```python
from build123d import *

# Parameters (mm, degrees)
PAD_DEPTH = 6


with BuildPart() as part:
    # Sketch → Pad (new body)
    with BuildSketch(Plane.XY):
        with BuildLine():
            ThreePointArc((-202.000023, 6.75), (-208.750028, -1e-06), (-202.000021, -6.75))
            Line((-202.000021, -6.75), (201.999979, -6.75))
            ThreePointArc((201.999979, -6.75), (208.74998, 1e-06), (201.999977, 6.75))
            Line((-202.000023, 6.75), (201.999977, 6.75))
        make_face()
        with BuildLine():
            Line((-202, 5.25), (202, 5.25))
            ThreePointArc((201.999976, -5.25), (207.24998, -1.2e-05), (202, 5.25))
            Line((201.999976, -5.25), (-202.000024, -5.25))
            ThreePointArc((-202, 5.25), (-207.250028, 1.2e-05), (-202.000024, -5.25))
        make_face(mode=Mode.SUBTRACT)
    extrude(amount=PAD_DEPTH)


solid = part.part
```
Model file for the job. Use its own axes, mm. Coordinates: 2 decimals unless noted, no trailing zeros. Loops run counter-clockwise (first coordinate to the right, second up) from the corner with the lowest first, then second, coordinate; pieces in that order, holes last. Notation, with made-up numbers: (9, 74) -> (57, 74) arc R5 ccw to (57, 82) -> close; hole circle Ø10 at (66, 13). An arc over 180 degrees is marked (long way). Answer as a JSON object with one key per item and string values.
Q1. Flat gauge pins, fed straight in: P1, Ø1, axis at y = 1.5, z = 1.5, coming from the -X side; P2, Ø1.5, axis at y = -0.5, z = 5, coming from the +X side. Where does each tip first touch, or does it go through?
Report:
{"P1": "stops at x = -208.68", "P2": "stops at x = 208.75"}
Q2. Cut at C-C (z = 4.55). List the corners of the cut face in (x, y).
Report:
{"outline": "(-202, -6.75) -> (202, -6.75) arc R6.75 ccw to (202, 6.75) -> (-202, 6.75) arc R6.75 ccw to start; hole (-202, -5.25) -> (202, -5.25) arc R5.25 ccw to (202, 5.25) -> (-202, 5.25) arc R5.25 ccw to start"}
Q3. Cut at B-B (y = -3). List the corners of the cut face in (x, z), and give its area (3 significant figures).
Report:
{"outline": "(-208.05, 0) -> (-206.31, 0) -> (-206.31, 6) -> (-208.05, 6) -> close; (206.31, 0) -> (208.05, 0) -> (208.05, 6) -> (206.31, 6) -> close", "area": "20.9 mm2"}
Q4. Probe probe 1 along Y at (x, z) = (106.5, 3.75); probe 2 along X at (y, z) = (0.5, 2.15). List the from-to ranges inside material, lowest first.
Report:
{"probe 1": "y = -6.75 to -5.25, 5.25 to 6.75", "probe 2": "x = -208.73 to -207.23, 207.23 to 208.73"}
Q5. Cut at A-A (x = 34.5). List the corners of the cut face in (y, z), and give its area (3 significant figures).
Report:
{"outline": "(-6.75, 0) -> (-5.25, 0) -> (-5.25, 6) -> (-6.75, 6) -> close; (5.25, 0) -> (6.75, 0) -> (6.75, 6) -> (5.25, 6) -> close", "area": "18.0 mm2"}
